Geometry check sheet. Reference: the model listing, model coordinates, mm. A direction names the side the tool comes from. Give positions to 0.01 mm unless a question says otherwise; leave off trailing zeros. Order: outer loops, then holes, each group sorted by start corner. A loop starts at its lowest first (then second) coordinate and runs counter-clockwise, first axis right, second up. Notation, with made-up numbers: M 42,-15.75 L 83,-15.75 A15 ccw 83,1.25 Z; hole C 36,50.5 d11. An arc over 180 degrees is marked long. Answer as CSV lines item,"result". Start each with the question number.
Q1. Section check D-D, the plane x = 32. Record the boundary of the cut face in (y, z), then the cut area to 3 significant figures.
Q2. Thickness scan on line 1 (X direction, y = 5, z = 5.75); line 2 (Z direction, x = 12, y = -6.5); line 3 (Y direction, x = 26.5, z = 4.3). Record the ranges inside material, lowest first.
Q3. Mould release check, pull along X, two halves, no side actions. Record for faces 6 (the flat face through (24, -5, 5)), 7 (the conical face through (14.14, 7.88, -7.72)), 8 (the conical face through (0.17, -5.83, 5.72)): +X half, -X half, draft (parallel to the pull), parting line (faces both ways), or undercut.
Q4. Section check A-A, the plane z = 0. Record the boundary of the cut face in (x, y), then the cut area to 3 significant figures.
Q5. Go/stop test with flat-tipped pins: pin 1 (2 mm diameter, centred on x = 11.5, y = -4.5, fed in from -Z); pin 2 (8 mm diameter, centred on x = 21, y = -3, fed in from +Z); pin 3 (3.5 mm diameter, centred on y = 7.5, z = 8.5, fed in from -X). Record where each tip stops, or that it passes through.
Q6. Set-up check for faces 1 (the cylindrical face through (26.5, 6, 2.5)), 2 (the flat face through (4, -7, 7)), 3 (the flat face through (4, 7, 7)), 4 (the flat face through (4, -7, -7)), 5 (the flat face through (13, -7, -1)): record each of +Z, -Z, +X, -X, +Y, -Y from which the full face is reachable in a straight line by a thin tool's end or side.
Q7. Section check C-C, the plane x = 27.5. Record the boundary of the cut face in (y, z), then the cut area to 3 significant figures.
```python
from build123d import *

# Parameters (mm, degrees)
CHAMFER_1_SIZE           = 1
SKETCH_2_R               = 1.5
CUT_EXTRUDE_1_DEPTH      = 40.210967853
SKETCH_3_W               = 30.067866829
SKETCH_3_H               = 2
CUT_EXTRUDE_1_2_DEPTH    = 40.210967853
PATTERN_CIRCULAR_1_COUNT = 4
CUT_EXTRUDE_2_DEPTH      = 40.185456486
CUT_EXTRUDE_2_DEPTH_BACK = 40.185456486
SKETCH_4_R               = 3.5


with BuildPart() as part:
    # 草图1 → 旋转1 (revolve)
    with BuildSketch(Plane.XY):
        Polygon((0, 0), (0, 9), (4, 9), (4, 12.5), (24, 9.60013801), (24, 6.5), (29, 6.5), (29, 9), (35, 9), (35, 0), align=None)
    revolve(axis=Axis((35, 0, 0), (-1, 0, 0)))

    # 倒角1
    chamfer_1_edges = [part.edges().sort_by_distance(p)[0] for p in [
        (0, -9, 0),
        (35, -9, 0),
    ]]
    chamfer(chamfer_1_edges, length=CHAMFER_1_SIZE)

    # 草图2 → Cut-Extrude 1 (cut, symmetric)
    with BuildSketch(Plane.XY):
        with Locations((26.5, 0)):
            Circle(SKETCH_2_R)
    cut_extrude_1 = extrude(amount=CUT_EXTRUDE_1_DEPTH, both=True, mode=Mode.SUBTRACT)

    # 草图3 → Cut-Extrude 1 2 (cut, symmetric)
    with BuildSketch(Plane.XY):
        with Locations((11.466066586, 0)):
            Rectangle(SKETCH_3_W, SKETCH_3_H)
    cut_extrude_1_2 = extrude(amount=CUT_EXTRUDE_1_2_DEPTH, both=True, mode=Mode.SUBTRACT)

    # 阵列(圆周)1: Cut-Extrude 1, Cut-Extrude 1 2 ×4 about axis
    pattern_circular_1_axis = Axis((35, 0, 0), (1, 0, 0))
    add([cut_extrude_1.rotate(pattern_circular_1_axis, i * 360 / PATTERN_CIRCULAR_1_COUNT) for i in range(1, PATTERN_CIRCULAR_1_COUNT)], mode=Mode.SUBTRACT)
    add([cut_extrude_1_2.rotate(pattern_circular_1_axis, i * 360 / PATTERN_CIRCULAR_1_COUNT) for i in range(1, PATTERN_CIRCULAR_1_COUNT)], mode=Mode.SUBTRACT)

    # 草图4 → 切除-拉伸2 (cut, two sides: drawn at the far end of the back side and taken through both)
    with BuildSketch(Plane(origin=(35, 0, 0), x_dir=(0, 0, -1), z_dir=(1, 0, 0)).offset(-CUT_EXTRUDE_2_DEPTH_BACK)):
        with Locations(Location((0, 0, 0), (0, 0, 90))):
            Circle(SKETCH_4_R)
    extrude(amount=CUT_EXTRUDE_2_DEPTH + CUT_EXTRUDE_2_DEPTH_BACK, mode=Mode.SUBTRACT)


solid = part.part
```
Answer block:
1,outline,"C 0,0 d18; hole C 0,0 d7"
1,area,"216 mm2"
2,line 1,"x = 0 to 24, 29 to 35"
2,line 2,"z = -9.29 to -1, 1 to 9.29"
2,line 3,"y = -4.87 to -1.5, 1.5 to 4.87"
3,face 6,"undercut"
3,face 7,"+X half"
3,face 8,"-X half"
4,outline,"M 28,-6.5 L 29,-6.5 L 29,-9 L 34,-9 L 35,-8 L 35,-3.5 L 28,-3.5 Z; M 28,3.5 L 35,3.5 L 35,8 L 34,9 L 29,9 L 29,6.5 L 28,6.5 Z"
4,area,"71.0 mm2"
5,pin 1,"stops at z = -10.9"
5,pin 2,"stops at z = 10.49"
5,pin 3,"stops at x = 4"
6,face 1,"none"
6,face 2,"+Z, -X, -Y"
6,face 3,"+Z, -X, +Y"
6,face 4,"-Z, -X, -Y"
6,face 5,"-X, +Y, -Y"
7,outline,"M -6.4,-1.12 A6.5 ccw -1.12,-6.4 L -1.12,-3.32 A3.5 cw -3.32,-1.12 Z; M -6.4,1.12 L -3.32,1.12 A3.5 cw -1.12,3.32 L -1.12,6.4 A6.5 ccw Z; M 1.12,-6.4 A6.5 ccw 6.4,-1.12 L 3.32,-1.12 A3.5 cw 1.12,-3.32 Z; M 1.12,3.32 A3.5 cw 3.32,1.12 L 6.4,1.12 A6.5 ccw 1.12,6.4 Z"
7,area,"67.2 mm2"
